Design review of the part shown in the three views and the two pictorial views. Dimensions are in mm from the part's minimum x, y and z. Coordinates: 2 decimals unless noted, no trailing zeros. Loops run counter-clockwise (first coordinate to the right, second up) from the corner with the lowest first, then second, coordinate; pieces in that order, holes last. Notation, with made-up numbers: M 61.5,-5 L 66.5,-5 A11 ccw 66.5,8 Z; hole C -21.5,50.5 d6. An arc over 180 degrees is marked long. Answer as a JSON object with one key per item and string values. Group by question number.
Item 1: Add section A-A (z = 101.6). State the section outline as (x, y) points, then the cut area to 3 significant figures.
Item 2: Add section D-D (z = 65.5). State the section outline as (x, y) points.
Item 3: Add section B-B (x = 101.6). State the section outline as (y, z) points.
Item 4: Insertion check: pin 1 (1 mm diameter, centred on y = 12, z = 56, fed in from +X); pin 2 (10 mm diameter, centred on y = 13, z = 129, fed in from -X); pin 3 (1 mm diameter, centred on x = 79, y = 7, fed in from +Z); pin 4 (4.5 mm diameter, centred on x = 162.09, z = 128.32, fed in from +Y). Each pin has a flat end and moves straight along its axis. Give the tip position at first contact, or say it passes through.
Item 5: Add section C-C (y = 7.5). Count the separate pieces of the cut face and the enclosed holes in it, then the cut area to 3 significant figures.
Item 6: Wall thickness on L1, parallel to X at y = 10, z = 147.5 (1 decimal); L2, parallel to Z at x = 99.5, y = 1.5; L3, parallel to X at y = 14, z = 107.5: over which ranges is each line inside the solid? List them lowest first. Write a range as from..to.
Item 7: Mouldability with a two-part tool opening along Z and no side actions: class the marked faces 1, 2 and 3 as +Z half, -Z half, draft (parallel to the pull), parting line (faces both ways), or undercut.
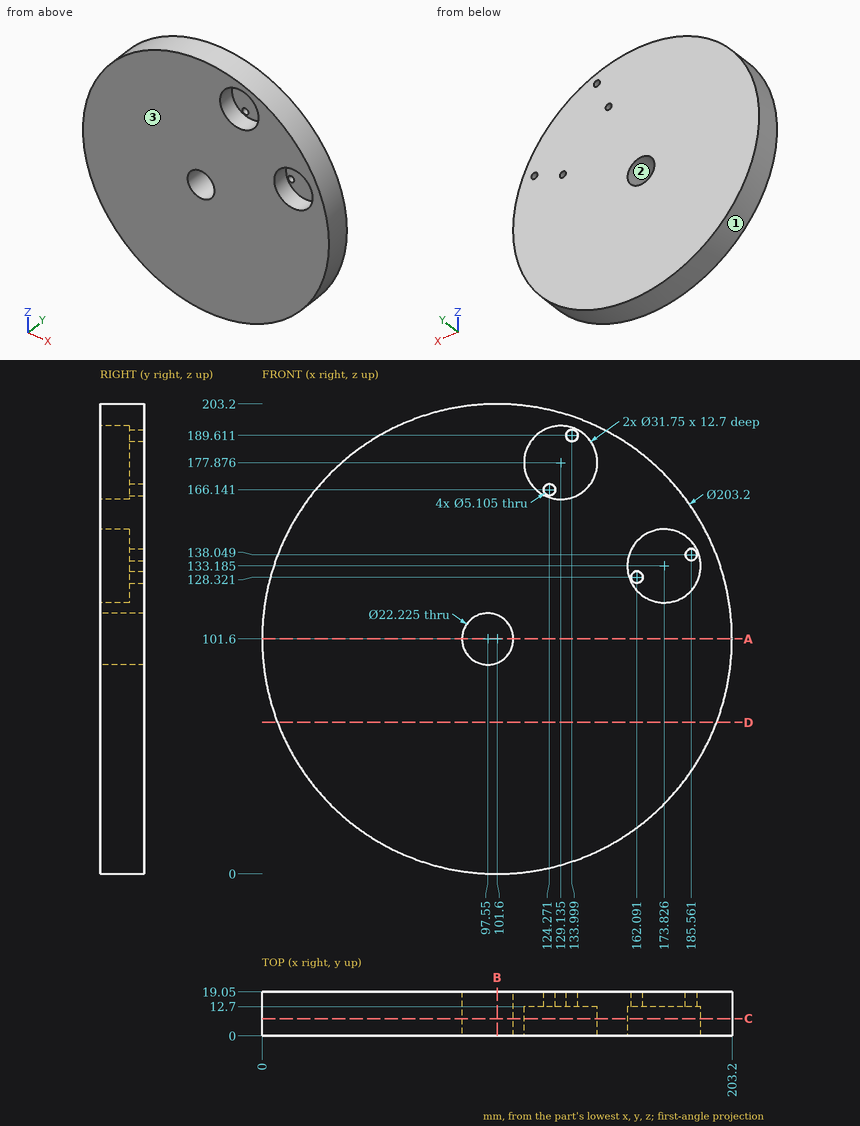
From the geometry:
{
 "1": {"outline": "M 0,0 L 86.44,0 L 86.44,19.05 L 0,19.05 Z; M 108.66,0 L 203.2,0 L 203.2,19.05 L 108.66,19.05 Z", "area": "3,450 mm²"},
 "2": {"outline": "M 6.63,0 L 196.57,0 L 196.57,19.05 L 6.63,19.05 Z"},
 "3": {"outline": "M 0,0 L 19.05,0 L 19.05,91.25 L 0,91.25 Z; M 0,111.95 L 19.05,111.95 L 19.05,203.2 L 0,203.2 Z"},
 "4": {"pin 1": "stops at x = 192.64", "pin 2": "stops at x = 2.5", "pin 3": "stops at z = 200.77", "pin 4": "passes through"},
 "5": {"separate pieces": "1", "enclosed holes": "3", "area": "30,500 mm²"},
 "6": {"L1": "x = 11..167, 180.7..192.2", "L2": "z = 0.02..90.66, 112.54..203.18", "L3": "x = 0.17..88.13, 106.97..203.03"},
 "7": {"face 1": "parting line", "face 2": "undercut", "face 3": "draft"}
}
